Input: part model. Units: mm. Frame: model coordinates. A direction names the side the tool comes from. Coordinates: 2 decimals unless noted, no trailing zeros. Write each loop counter-clockwise with the first axis right and the second up, starting at its lowest first coordinate (ties: lowest second). Pieces come first, ordered by that corner, then holes. Notation, with made-up numbers: (14, -11.5) -> (22, -11.5) arc R22 cw to (22, 9.5) -> close; hole circle Ø9 at (81.25, 31.5). An arc over 180 degrees is marked (long way). One line per question, with ' | ' between items. Start each with the question number.
```python
from build123d import *

# Parameters (mm, degrees)
F0_W     = 20
F0_H     = 20
F1_DEPTH = 10
F1_TAPER = 3
F2_R     = 3
F3_W     = 7.29034096
F3_H     = 8.2890868653
F4_DEPTH = 2


with BuildPart() as f1:
    # F0 (on Top) → F1 (new body)
    with BuildSketch(Plane.XY):
        with Locations((0, -0.8712120694)):
            Rectangle(F0_W, F0_H)
    extrude(amount=F1_DEPTH, taper=F1_TAPER)

    # F2
    f2_edges = [f1.edges().sort_by_distance(p)[0] for p in [
        (0, 8.60471, 10),
        (-9.737961, 8.866749, 5),
        (-9.475922, -0.871212, 10),
        (-9.737961, -10.609173, 5),
        (0, -10.347134, 10),
        (9.475922, -0.871212, 10),
        (9.737961, 8.866749, 5),
        (9.737961, -10.609173, 5),
    ]]
    fillet(f2_edges, radius=F2_R)

    # F3 (on face) → F4 (cut)
    with BuildSketch(Plane.XY.offset(10)):
        with Locations((0.0642689411, -0.9792846395)):
            Rectangle(F3_W, F3_H)
    extrude(amount=-F4_DEPTH, mode=Mode.SUBTRACT)


solid = f1.part
```
1) Access query for faces 1 (the face through (-8.72, -0.96, 9.15)), 2 (the face through (0, 3.165, 9)). Directions: +Z, -Z, +X, -X, +Y, -Y. A direction counts if a zero-diameter tool reaches every point of the face in a straight line with its end or side. Return the directions, or none.
2) Section D-D, the plane z = 8.75. Return loops of the section in (x, y), then the cut area to 3 significant figures.
3) Section A-A, the plane y = 1.75. Return loops of the section in (x, z), then the cut area to 3 significant figures.
4) Section C-C, the plane z = 7.5. Return loops of the section in (x, y).
5) First-contact query: P1, Ø2, axis at x = -1, z = 9, coming from the -Y side; P2, Ø1, axis at y = 0, z = 6, coming from the -X side; P3, Ø0.6, axis at y = -0.5, z = 9, coming from the -X side. Flat tips, straight axial feed; report the tip coordinate or a pass-through.
6) Pull-direction query (X, two-part tool) for faces 3 (the face through (0, -5.124, 9)), 4 (the face through (3.709, -1, 9)), 5 (the face through (-0.098, 8.944, 3.528)), 6 (the face through (8.72, -0.78, 9.15)); classes: released by +X, released by -X, zero draft, split by the parting line, or undercut.
7) Ray query, line 1 (X direction, y = -6, z = 7.25); line 2 (Y direction, x = 0.75, z = 9); line 3 (Z direction, x = 6.75, y = -6.25). Return the intervals inside material, ascending.
8) Section B-B, the plane x = 1.5. Return loops of the section in (y, z), then the cut area to 3 significant figures.
Answer block:
1) face 1: +Z, -X, +Y, -Y | face 2: +Z
2) outline: (-9.07, -7.5) arc R2.44 ccw to (-6.63, -9.94) -> (6.63, -9.94) arc R2.44 ccw to (9.07, -7.5) -> (9.07, 5.76) arc R2.44 ccw to (6.63, 8.19) -> (-6.63, 8.19) arc R2.44 ccw to (-9.07, 5.76) -> close; hole (-3.58, -5.12) -> (3.71, -5.12) -> (3.71, 3.17) -> (-3.58, 3.17) -> close | area: 263 mm2
3) outline: (-10, 0) -> (10, 0) -> (9.62, 7.16) arc R3 ccw to (6.63, 10) -> (3.71, 10) -> (3.71, 8) -> (-3.58, 8) -> (-3.58, 10) -> (-6.63, 10) arc R3 ccw to (-9.62, 7.16) -> close | area: 177 mm2
4) outline: (-9.59, -7.5) arc R2.96 ccw to (-6.63, -10.46) -> (6.63, -10.46) arc R2.96 ccw to (9.59, -7.5) -> (9.59, 5.76) arc R2.96 ccw to (6.63, 8.72) -> (-6.63, 8.72) arc R2.96 ccw to (-9.59, 5.76) -> close
5) P1: stops at y = -10.33 | P2: stops at x = -9.71 | P3: stops at x = -9.1
6) face 3: undercut | face 4: undercut | face 5: zero draft | face 6: released by +X
7) line 1: x = -9.62 to 9.62 | line 2: y = -9.74 to -5.12, 3.17 to 7.99 | line 3: z = 0 to 10
8) outline: (-10.87, 0) -> (9.13, 0) -> (8.75, 7.16) arc R3 ccw to (5.76, 10) -> (3.17, 10) -> (3.17, 8) -> (-5.12, 8) -> (-5.12, 10) -> (-7.5, 10) arc R3 ccw to (-10.5, 7.16) -> close | area: 175 mm2
